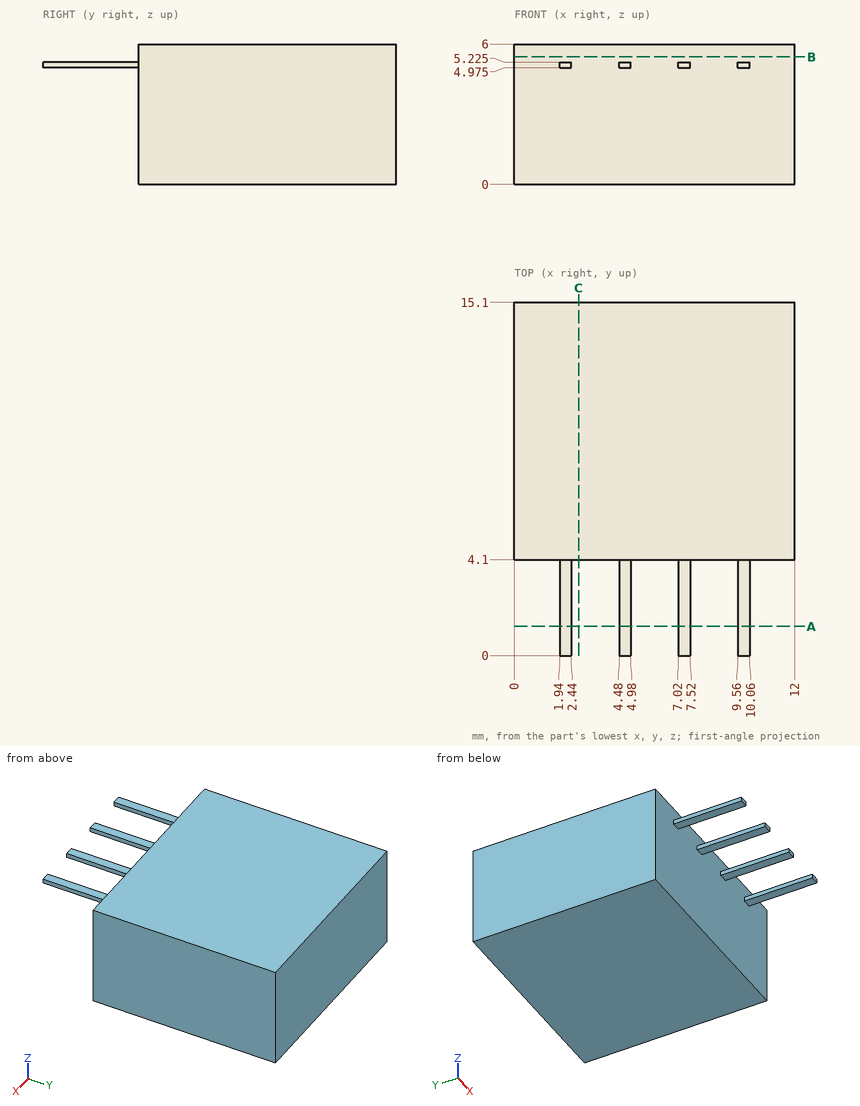
Here's the drawing with two shaded views (mm, measured from the low corner). I have some questions. Round coordinates to 2 decimals unless told otherwise and drop trailing zeros. Loops run counter-clockwise (first coordinate to the right, second up) from the corner with the lowest first, then second, coordinate; pieces in that order, holes last. Notation, with made-up numbers: (-21.5, 50) - (29.5, 50) arc R28 cw to (29.5, 77) - close; hole circle Ø7 at (-11.75, 27.5). An arc over 180 degrees is marked (long way). Write item = value, one per line.
1) Imagine slicing it at C-C (x = 2.75). Please give me the cut outline in (y, z), and give its area (3 significant figures).
Computed:
outline = (4.1, 0) - (15.1, 0) - (15.1, 6) - (4.1, 6) - close
area = 66.0 mm2
2) Imagine slicing it at A-A (y = 1.25). Please give me the cut outline in (x, z) (3 decimals).
Computed:
outline = (1.94, 4.975) - (2.44, 4.975) - (2.44, 5.225) - (1.94, 5.225) - close; (4.48, 4.975) - (4.98, 4.975) - (4.98, 5.225) - (4.48, 5.225) - close; (7.02, 4.975) - (7.52, 4.975) - (7.52, 5.225) - (7.02, 5.225) - close; (9.56, 4.975) - (10.06, 4.975) - (10.06, 5.225) - (9.56, 5.225) - close
3) I need wall thicknesses on line 1 along X through (y, z) = (1.5, 5.05); line 2 along Y through (x, z) = (10, 4.25). Which ranges of each line are inside material? Lowest first, please. Write a range as from..to.
Computed:
line_1 = 1.94..2.44, 4.48..4.98, 7.02..7.52, 9.56..10.06
line_2 = 4.1..15.1
4) I'm going to push flat-ended pins straight in: P1, Ø0.6, axis at x = 2.5, y = 1.5, coming from the -Z side (3 decimals); P2, Ø3, axis at x = 9, z = 1, coming from the -Y side. Where does each tip first touch, or does it pass through?
Computed:
P1 = 4.975
P2 = 4.1
5) Imagine slicing it at B-B (z = 5.45). Please give me the cut outline in (x, y).
Computed:
outline = (0, 4.1) - (12, 4.1) - (12, 15.1) - (0, 15.1) - close
